Can you work these out from the drawing? Everything is in mm from the part's minimum corner. A direction names the side the tool comes from. Coordinates: 2 decimals unless noted, no trailing zeros. Order: outer loops, then holes, each group sorted by start corner. A loop starts at its lowest first (then second) coordinate and runs counter-clockwise, first axis right, second up. Notation, with made-up numbers: (-36.5, 67) -> (-23.5, 67) arc R22 cw to (-23.5, 100) -> close; hole circle Ø7 at (0.25, -35.75). An arc over 180 degrees is marked (long way). Write item = value, one per line. Start each with the question number.
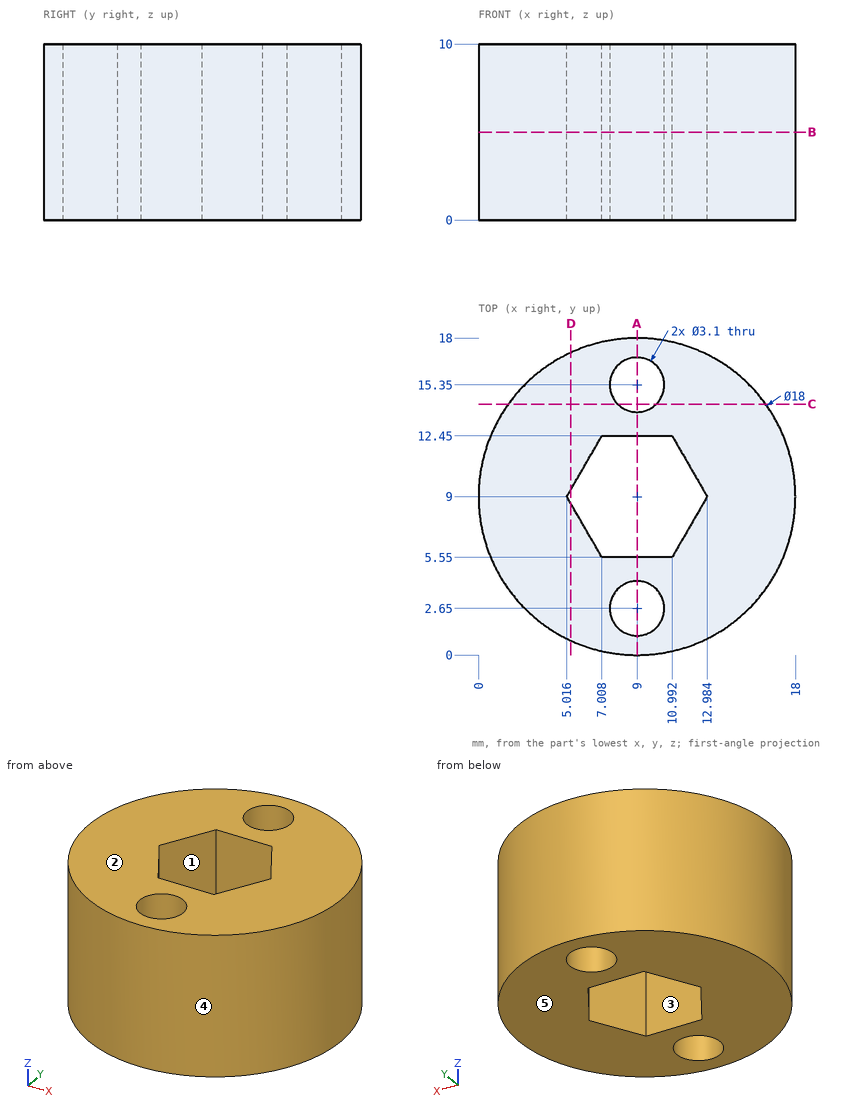
(1) Imagine slicing it at A-A (x = 9). Write out the boundary of the cut face in (y, z).
(2) For the marked faces 1 and 2, which set-ups out of +Z, -Z, +X, -X, +Y, -Y let a thin tool reach every point of the face, with its end or its side?
(3) Imagine slicing it at B-B (z = 5). Write out the boundary of the cut face in (x, y), plus the area to 3 significant figures.
(4) Thinking about a two-plate mould opening in Y: for the marked faces 3, 4 and 5, which applies, +Y half, -Y half, draft (parallel to the pull), parting line (faces both ways), or undercut?
(5) For P1, Ø1, axis at y = 5.5, z = 3.5, coming from the +X side (1 decimal); P2, Ø1.5, axis at x = 12.5, z = 2, coming from the -Y side; P3, Ø1.9, axis at x = 9, y = 2.65, coming from the -Z side; P4, Ø3, axis at y = 15.5, z = 5, coming from the -X side, each with a flat end and sliding along its axis, tell me the tip position at first contact or that it passes through.
(6) If I drill on L1, parallel to Y at x = 9, z = 5; L2, parallel to Y at x = 6.75, z = 1 (1 decimal); L3, parallel to X at y = 10.25, z = 7, over which ranges is the centre line in solid material (lowest first)? Write a range as from..to.
(7) Imagine slicing it at C-C (y = 14.25). Write out the boundary of the cut face in (x, z), plus the area to 3 significant figures.
(8) Imagine slicing it at D-D (x = 5.25). Write out the boundary of the cut face in (y, z) (1 decimal).
Result set:
q1.outline = (0, 0) -> (1.1, 0) -> (1.1, 10) -> (0, 10) -> close; (4.2, 0) -> (5.55, 0) -> (5.55, 10) -> (4.2, 10) -> close; (12.45, 0) -> (13.8, 0) -> (13.8, 10) -> (12.45, 10) -> close; (16.9, 0) -> (18, 0) -> (18, 10) -> (16.9, 10) -> close
q2.face_1 = +Z, -Z
q2.face_2 = +Z, +X, -X, +Y, -Y
q3.outline = circle Ø18 at (9, 9); hole (5.02, 9) -> (7.01, 5.55) -> (10.99, 5.55) -> (12.98, 9) -> (10.99, 12.45) -> (7.01, 12.45) -> close; hole circle Ø3.1 at (9, 2.65); hole circle Ø3.1 at (9, 15.35)
q3.area = 198 mm2
q4.face_3 = undercut
q4.face_4 = parting line
q4.face_5 = draft
q5.P1 = 17.5
q5.P2 = 0.43
q5.P3 = through
q5.P4 = 1.52
q6.L1 = 0..1.1, 4.2..5.55, 12.45..13.8, 16.9..18
q6.L2 = 0.3..6, 12..17.7
q6.L3 = 0.09..5.74, 12.26..17.91
q7.outline = (1.69, 0) -> (7.91, 0) -> (7.91, 10) -> (1.69, 10) -> close; (10.09, 0) -> (16.31, 0) -> (16.31, 10) -> (10.09, 10) -> close
q7.area = 124 mm2
q8.outline = (0.8, 0) -> (8.6, 0) -> (8.6, 10) -> (0.8, 10) -> close; (9.4, 0) -> (17.2, 0) -> (17.2, 10) -> (9.4, 10) -> close
